Verification items for the finished model (mm, model axes). Face numbers are marked on the shaded views. Give positions to 0.01 mm unless a question says otherwise; leave off trailing zeros. Loops run counter-clockwise (first coordinate to the right, second up) from the corner with the lowest first, then second, coordinate; pieces in that order, holes last. Notation, with made-up numbers: (37, 81.25) - (45, 81.25) arc R27 ccw to (45, 117.25) - close; hole circle Ø5 at (65, 81.5). An arc over 180 degrees is marked (long way). Put each result on its own line as item: value. Start each with the question number.
```python
from build123d import *

# Parameters (mm, degrees)
SKETCH1_R           = 2
SKETCH1_R_2         = 8
BOSS_EXTRUDE1_DEPTH = 7


with BuildPart() as part:
    # Sketch1 → Boss-Extrude1 (new, symmetric)
    with BuildSketch(Plane.XY):
        with BuildLine():
            Line((-30, 9), (30, 9))
            ThreePointArc((30, 9), (39, 0), (30, -9))
            Line((30, -9), (-30, -9))
            ThreePointArc((-30, -9), (-39, 0), (-30, 9))
        make_face()
        with Locations((-15, 0)):
            Circle(SKETCH1_R, mode=Mode.SUBTRACT)
        with Locations((15, 0)):
            Circle(SKETCH1_R, mode=Mode.SUBTRACT)
        with Locations((-30, 0)):
            Circle(SKETCH1_R_2, mode=Mode.SUBTRACT)
        with Locations((30, 0)):
            Circle(SKETCH1_R_2, mode=Mode.SUBTRACT)
    extrude(amount=BOSS_EXTRUDE1_DEPTH, both=True)


solid = part.part
```
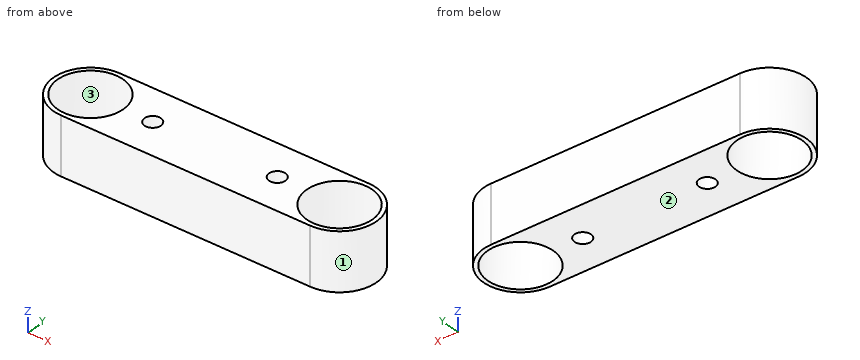
1) Scan lines: line 1 along X through (y, z) = (5.25, -1); line 2 along X through (y, z) = (-5, -3) (3 decimals); line 3 along Y through (x, z) = (15, 0.75). Record each from-to range of solid material in increasing order. Write a range as from..to.
2) Section check B-B, the plane y = 0. Enter the section's corners in (x, z), plus the area to 3 significant figures.
3) Section check A-A, the plane x = 15. Enter the section's corners in (y, z), plus the area to 3 significant figures.
4) Draft check along X on the marked faces 1, 2 and 3. Enter one of: pulls with the +X half, pulls with the -X half, needs draft (parallel to the pull), parting line crosses it, or undercut.
5) Section check C-C, the plane z = 0.75. Enter the section's corners in (x, y).
6) Section check D-D, the plane y = 6. Enter the section's corners in (x, z).
Results are:
1. line 1: x = -37.31..-36.04, -23.96..23.96, 36.04..37.31
1. line 2: x = -37.483..-36.245, -23.755..23.755, 36.245..37.483
1. line 3: y = -9..-2, 2..9
2. outline: (-39, -7) - (-38, -7) - (-38, 7) - (-39, 7) - close; (-22, -7) - (-17, -7) - (-17, 7) - (-22, 7) - close; (-13, -7) - (13, -7) - (13, 7) - (-13, 7) - close; (17, -7) - (22, -7) - (22, 7) - (17, 7) - close; (38, -7) - (39, -7) - (39, 7) - (38, 7) - close
2. area: 532 mm2
3. outline: (-9, -7) - (-2, -7) - (-2, 7) - (-9, 7) - close; (2, -7) - (9, -7) - (9, 7) - (2, 7) - close
3. area: 196 mm2
4. face 1: pulls with the +X half
4. face 2: needs draft
4. face 3: undercut
5. outline: (-30, -9) - (30, -9) arc R9 ccw to (30, 9) - (-30, 9) arc R9 ccw to start; hole circle Ø16 at (-30, 0); hole circle Ø4 at (-15, 0); hole circle Ø4 at (15, 0); hole circle Ø16 at (30, 0)
6. outline: (-36.71, -7) - (-35.29, -7) - (-35.29, 7) - (-36.71, 7) - close; (-24.71, -7) - (24.71, -7) - (24.71, 7) - (-24.71, 7) - close; (35.29, -7) - (36.71, -7) - (36.71, 7) - (35.29, 7) - close
